```python
from build123d import *

# Parameters (mm, degrees)
SKETCH1_W                 = 150
SKETCH1_H                 = 80
BOSS_EXTRUDE1_DEPTH       = 60
SHELL1_T                  = -5
SHELL1_THICKNESS_2_FACE_W = 75
SHELL1_THICKNESS_2_FACE_H = 140
SHELL1_THICKNESS_2_DEPTH  = 5


with BuildPart() as part:
    # Sketch1 → Boss-Extrude1 (new body)
    with BuildSketch(Plane(origin=(0, 0, 0), x_dir=(1, 0, 0), z_dir=(0, 1, 0))):
        with Locations((75, 40)):
            Rectangle(SKETCH1_W, SKETCH1_H)
    extrude(amount=BOSS_EXTRUDE1_DEPTH)

    # Shell1
    shell1_openings = [part.faces().sort_by_distance(p)[0] for p in [
        (75, 30, 0),
    ]]
    offset(amount=SHELL1_T, openings=shell1_openings, kind=Kind.INTERSECTION)

    # Shell1 thickness 2 face (on inner face of the shell) → Shell1 thickness 2 (add)
    with BuildSketch(Plane(origin=(75, 55, -37.5), x_dir=(0, 0, 1), z_dir=(0, 1, 0))):
        Rectangle(SHELL1_THICKNESS_2_FACE_W, SHELL1_THICKNESS_2_FACE_H)
    extrude(amount=-SHELL1_THICKNESS_2_DEPTH)


solid = part.part
```
Input: part model. Units: mm. Frame: model coordinates. A direction names the side the tool comes from. Give positions to 0.01 mm unless a question says otherwise; leave off trailing zeros. Order: outer loops, then holes, each group sorted by start corner. A loop starts at its lowest first (then second) coordinate and runs counter-clockwise, first axis right, second up.
1. Cut plane B-B (y = 45). Return loops of the section in (x, z), and give its area (3 significant figures).
Computed:
outline: (0, -80) - (150, -80) - (150, 0) - (145, 0) - (145, -75) - (5, -75) - (5, 0) - (0, 0) - close
area: 1,500 mm2
2. Pin query (flat end, axial travel): pin 1 Ø1.5 at (x, y) = (15.5, 8) entering from +Z. Return the tip coordinate at first contact, or that it passes through.
Computed:
pin 1: stops at z = -75
3. Cut plane A-A (z = -25). Return loops of the section in (x, y), and give its area (3 significant figures).
Computed:
outline: (0, 0) - (150, 0) - (150, 60) - (0, 60) - close; hole (5, 5) - (145, 5) - (145, 50) - (5, 50) - close
area: 2,700 mm2
4. Line query: probe 1 along X at (y, z) = (12, -61); probe 2 along Y at (x, z) = (117, -15.5); probe 3 along Z at (x, y) = (127, 43). Output: solid intervals per line, ascending.
Computed:
probe 1: x = 0 to 5, 145 to 150
probe 2: y = 0 to 5, 50 to 60
probe 3: z = -80 to -75
5. Set-up query: faces 1 (the face through (5, 27, -37)), 2 (the face through (74, 0, -41)). Return all of +Z, -Z, +X, -X, +Y, -Y with unobstructed straight access to the full face (end or side cutting, diameter ignored); none if empty.
Computed:
face 1: +Z
face 2: +Z, -Z, +X, -X, -Y
6. Cut plane C-C (x = 84.5). Return loops of the section in (y, z), and give its area (4 significant figures).
Computed:
outline: (0, -80) - (60, -80) - (60, 0) - (50, 0) - (50, -75) - (5, -75) - (5, 0) - (0, 0) - close
area: 1,425 mm2
7. Draft query along X for faces 3 (the face through (74, 5, -38)), 4 (the face through (0, 30, -39)), 5 (the face through (69, 52, 0)). Return one class per face: released by +X, released by -X, zero draft, split by the parting line, or undercut.
Computed:
face 3: undercut
face 4: released by -X
face 5: zero draft
